from build123d import *

# Parameters (mm, degrees)
SKETCH2_R                     = 19.0875
BOSS_EXTRUDE1_DEPTH           = 100
BOSS_EXTRUDE2_REACH           = 96.162
BOSS_EXTRUDE2_END_RADIUS      = 19.0875
SKETCH3_R                     = 19.0875
SHELL1_OUTLINE_R              = 17.0875
SHELL1_DEPTH                  = 100
SHELL1_START                  = -37.059047745
SHELL1_2_OUTLINE_R            = 17.0875
SHELL1_2_DEPTH                = 50.0000001
SKETCH8_R                     = 17.0875
SKETCH8_R_2                   = 12.7
BOSS_EXTRUDE3_DEPTH           = 100
SKETCH6_W                     = 2.75
SKETCH6_H                     = 19.0875
M5_CLEARANCE_HOLE1_AT_2_COUNT = 2
M5_CLEARANCE_HOLE1_AT_2_PITCH = 55.53473382
MIRROR1_COPY_1_SKETCH_W       = 2.75
MIRROR1_COPY_1_SKETCH_H       = 19.0875


with BuildPart() as part:
    # Sketch2 → Boss-Extrude1 (new body)
    with BuildSketch(Plane(origin=(0, 0, 0), x_dir=(0, 0, -1), z_dir=(1, 0, 0))):
        Circle(SKETCH2_R)
    extrude(amount=BOSS_EXTRUDE1_DEPTH)

    # Boss-Extrude2: up to this cylinder (the profile starts outside it)
    boss_extrude2_end = Plane(origin=(37.059048, 0, 0), z_dir=(-1, 0, 0)) * Cylinder(BOSS_EXTRUDE2_END_RADIUS, 231.499, mode=Mode.PRIVATE)
    # Sketch3 → Boss-Extrude2 (add, up to the surface)
    with BuildSketch(Plane(origin=(37.059047745, 0, 48.296291314), x_dir=(0.9659258262890673, 0, 0.2588190451025246), z_dir=(-0.2588190451025246, 0, 0.9659258262890673)), mode=Mode.PRIVATE) as boss_extrude2_sk1:
        Circle(SKETCH3_R)
    boss_extrude2_tool1 = extrude(boss_extrude2_sk1.sketch, amount=-BOSS_EXTRUDE2_REACH, mode=Mode.PRIVATE) - boss_extrude2_end
    add(boss_extrude2_tool1.solids().sort_by_distance((37.059048, 0, 48.296291))[0])

    # Shell1: read off the stored shape, not the designer's step
    # Shell1 outline → Shell1 (cut)
    with BuildSketch(Plane.YZ):
        Circle(SHELL1_OUTLINE_R)
    extrude(amount=SHELL1_DEPTH, mode=Mode.SUBTRACT)

    # Shell1 2 outline → Shell1 2 (cut)
    with BuildSketch(Plane(origin=(0, 0, 0), x_dir=(0.9659258262890672, 0, 0.2588190451025251), z_dir=(0.25881904510252507, 0, -0.9659258262890672)).offset(SHELL1_START)):
        with Locations((48.296291314, 0)):
            Circle(SHELL1_2_OUTLINE_R)
    extrude(amount=SHELL1_2_DEPTH, mode=Mode.SUBTRACT)

    # Sketch8 → Boss-Extrude3 (add, through all)
    with BuildSketch(Plane(origin=(100, 0, 0), x_dir=(0, 0, -1), z_dir=(1, 0, 0))):
        Circle(SKETCH8_R)
        Circle(SKETCH8_R_2, mode=Mode.SUBTRACT)
    extrude(amount=-BOSS_EXTRUDE3_DEPTH)

    # Sketch6 → M5 Clearance Hole1 (revolve, cut)
    with BuildSketch(Plane(origin=(85, 0, 0), x_dir=(0, 0, -1), z_dir=(1, 0, 0))):
        with Locations((1.375, 9.54375)):
            Rectangle(SKETCH6_W, SKETCH6_H)
    m5_clearance_hole1 = revolve(axis=Axis((85, -6.35, 0), (0, 1, 0)), mode=Mode.SUBTRACT)

    # M5 Clearance Hole1 at 2: M5 Clearance Hole1 ×2
    with Locations(*[Vector(-0.7933533402912365, 0, 0.608761429008719) * (i * M5_CLEARANCE_HOLE1_AT_2_PITCH) for i in range(1, M5_CLEARANCE_HOLE1_AT_2_COUNT)]):
        add(m5_clearance_hole1, mode=Mode.SUBTRACT)

    # Mirror1: M5 Clearance Hole1 across plane
    add(m5_clearance_hole1.mirror(Plane.ZX), mode=Mode.SUBTRACT)

    # Mirror1 copy 1 sketch → Mirror1 copy 1 (revolve, cut)
    with BuildSketch(Plane(origin=(40.941333421, 0, 33.80740392), x_dir=(0, 0, -1), z_dir=(1, 0, 0))):
        with Locations((1.375, -9.54375)):
            Rectangle(MIRROR1_COPY_1_SKETCH_W, MIRROR1_COPY_1_SKETCH_H)
    revolve(axis=Axis((40.941333421, 6.35, 33.80740392), (0, 1, 0)), mode=Mode.SUBTRACT)


solid = part.part
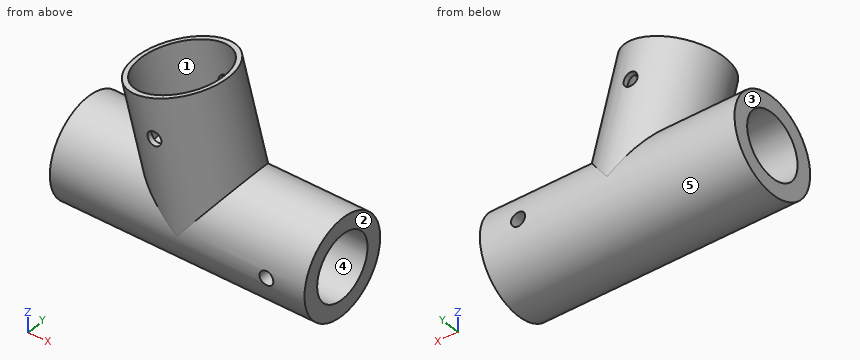
Could you check a few things on this model? Use its own coordinates, in mm. Face numbers are marked on the shaded views. A direction names the side the tool comes from. Coordinates: 2 decimals unless noted, no trailing zeros. Write each loop counter-clockwise with the first axis right and the second up, starting at its lowest first coordinate (ties: lowest second). Pieces come first, ordered by that corner, then holes. Notation, with made-up numbers: M 20.5,16 L 46.5,16 A24 cw 46.5,33 Z; hole C 78.25,65.25 d10. An arc over 180 degrees is marked long. One line per question, with ' | ' between items.
1) For pin 1 Ø2 at (x, y) = (43.5, -9) entering from -Z; pin 2 Ø3 at (y, z) = (-8.5, 42) entering from +X; pin 3 Ø12 at (y, z) = (-14.5, 30) entering from +X; pin 4 Ø3.5 at (x, z) = (40.94, 33.81) entering from +Y, each with a flat end and sliding along its axis, tell me the tip position at first contact or that it passes through.
Checks:
pin 1: z = -17.33 | pin 2: x = 57.25 | pin 3: x = 60.03 | pin 4: through
2) I need wall thicknesses on probe 1 along X at (y, z) = (-14, 0); probe 2 along Y at (x, z) = (78, 0); probe 3 along Z at (x, y) = (69.5, -6). Which ranges of each line are inside material? Lowest first, please. Write a range as [from, to].
Checks:
probe 1: [0, 82.25], [87.75, 100] | probe 2: [-19.09, -12.7], [12.7, 19.09] | probe 3: [-18.12, -11.19], [11.19, 18.12]
3) Imagine slicing it at D-D, the plane y = -14.5. Write out the boundary of the cut face in (x, z), and give its area (3 significant figures).
Checks:
outline: M 0,-12.41 L 100,-12.41 L 100,12.41 L 59.52,12.41 L 49.05,51.51 L 45.79,50.64 L 56.94,9.04 L 38.22,9.04 L 28.33,45.96 L 25.07,45.08 L 33.82,12.41 L 0,12.41 Z; hole C 85,0 d5.5 | area: 2,650 mm²
4) Imagine slicing it at B-B, the plane z = -7.5. Write out the boundary of the cut face in (x, y).
Checks:
outline: M 0,-17.55 L 100,-17.55 L 100,-10.25 L 0,-10.25 Z; M 0,10.25 L 100,10.25 L 100,17.55 L 0,17.55 Z
5) If we mould it in two halves opening along X, with no side actions, what happens to the marked faces 1, 2 and 3? For each: released by +X, released by -X, zero draft, split by the parting line, or undercut.
Checks:
face 1: undercut | face 2: released by +X | face 3: released by -X
6) For the marked faces 4 and 5, which set-ups out of +Z, -Z, +X, -X, +Y, -Y let a thin tool reach every point of the face, with its end or its side?
Checks:
face 4: +X, -X | face 5: none
7) Imagine slicing it at A-A, the plane y = 0. Write out the boundary of the cut face in (x, z).
Checks:
outline: M 0,-19.09 L 100,-19.09 L 100,-12.7 L 0,-12.7 Z; M 0,12.7 L 100,12.7 L 100,19.09 L 64.65,19.09 L 55.5,53.24 L 53.56,52.72 L 63.11,17.09 L 27.73,17.09 L 20.55,43.87 L 18.62,43.36 L 25.12,19.09 L 0,19.09 Z
